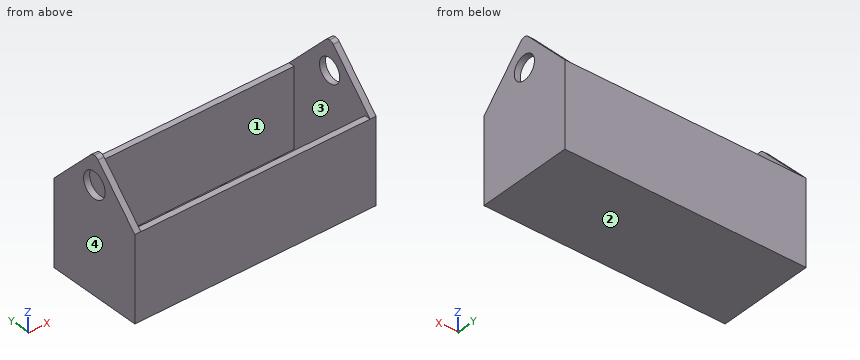
from build123d import *

# Parameters (mm, degrees)
F0_W      = 254
F0_H      = 101.6
F1_DEPTH  = 88.9
F4_DEPTH  = 6.35
F2_W      = 241.3
F2_H      = 88.9
F8_DEPTH  = 82.55
F9_R      = 12.7
F10_DEPTH = 25.4
F11_R     = 13.5154213428
F12_DEPTH = 25.4


with BuildPart() as f1:
    # F0 (on Top) → F1 (new body)
    with BuildSketch(Plane.XY):
        with Locations((77.3512227356, 27.0002914594)):
            Rectangle(F0_W, F0_H)
    extrude(amount=F1_DEPTH)

    # F3 (on face) → F4 (join)
    with BuildSketch(Plane.YZ.offset(204.3512227356)):
        with BuildLine():
            Line((22.3877730248, 137.7143067824), (-23.7997085406, 88.9))
            Line((-23.7997085406, 88.9), (27.0002914594, 88.9))
            Line((27.0002914594, 88.9), (27.0002914594, 139.7))
            ThreePointArc((27.0002914594, 139.7), (24.489399991, 139.1824886656), (22.3877730248, 137.7143067824))
        make_face()
        with BuildLine():
            Line((27.0002914594, 139.7), (27.0002914594, 88.9))
            Line((27.0002914594, 88.9), (77.8002914594, 88.9))
            Line((77.8002914594, 88.9), (31.6128098939, 137.7143067824))
            ThreePointArc((31.6128098939, 137.7143067824), (29.5111829277, 139.1824886656), (27.0002914594, 139.7))
        make_face()
    extrude(amount=-F4_DEPTH)

    # F7: F1 across plane


with BuildPart() as f1_1:
    add(f1.part)
    add(f1.part.mirror(Plane(origin=(77.3512227356, 27.0002914594, 88.9), x_dir=(0, 1, 0), z_dir=(1, 0, 0))))

    # F2 (on face) → F8 (cut)
    with BuildSketch(Plane.XY.offset(88.9)):
        with Locations((77.3512227356, 27.0002914594)):
            Rectangle(F2_W, F2_H)
    extrude(amount=-F8_DEPTH, mode=Mode.SUBTRACT)

    # F9 (on face) → F10 (cut)
    with BuildSketch(Plane.YZ.offset(204.3512227356)):
        with Locations((27.0002914594, 109.2127263546)):
            Circle(F9_R)
    extrude(amount=-F10_DEPTH, mode=Mode.SUBTRACT)

    # F11 (on face) → F12 (cut)
    with BuildSketch(Plane(origin=(-49.6487772644, 0, 0), x_dir=(0, -1, 0), z_dir=(-1, 0, 0))):
        with Locations((-27.0002914594, 110.0281476974)):
            Circle(F11_R)
    extrude(amount=-F12_DEPTH, mode=Mode.SUBTRACT)


solid = f1_1.part
Could you check a few things on this model? Use its own coordinates, in mm. Face numbers are marked on the shaded views. Give positions to 0.01 mm unless a question says otherwise; leave off trailing zeros. Order: outer loops, then holes, each group sorted by start corner. A loop starts at its lowest first (then second) coordinate and runs counter-clockwise, first axis right, second up. Notation, with made-up numbers: (69, 81) - (95, 81) arc R21 cw to (95, 120) - close; hole circle Ø5 at (-26, 60). An arc over 180 degrees is marked (long way). Return JSON: item names as keys, results as strings. Group by question number.
Q1. Suppose I cut it at B-B, the plane z = 99.5. Please give me the cut outline in (x, y), and give its area (3 significant figures).
Q2. Suppose I cut it at A-A, the plane z = 42.5. Please give me the cut outline in (x, y).
Q3. Suppose I cut it at D-D, the plane x = 182. Please give me the cut outline in (y, z), and give its area (3 significant figures).
Q4. Will these pins go through, and if not, where does the flat tip stop? pin 1 Ø1 at (x, y) = (53.5, -8) entering from +Z; pin 2 Ø1.9 at (x, y) = (121.5, 73) entering from +Z.
Q5. Suppose I cut it at C-C, the plane y = -8. Please give me the cut outline in (x, z), and give its area (3 significant figures).
Q6. Thinking about a two-plate mould opening in X: for the marked faces 1, 2, 3 and 4, which applies, pulls with the +X half, pulls with the -X half, needs draft (parallel to the pull), parting line crosses it, or undercut?
Q7. Please list where these lines run through material, in increasing order: line 1 along X through (y, z) = (32, 77.5); line 2 along Y through (x, z) = (164, 87); line 3 along Z through (x, y) = (94.5, 27.5). Write a range as [from, to].
Resolved:
{
 "1": {"outline": "(-49.65, -13.77) - (-43.3, -13.77) - (-43.3, 18.53) - (-49.65, 18.53) - close; (-49.65, 35.48) - (-43.3, 35.48) - (-43.3, 67.77) - (-49.65, 67.77) - close; (198, -13.77) - (204.35, -13.77) - (204.35, 18.82) - (198, 18.82) - close; (198, 35.18) - (204.35, 35.18) - (204.35, 67.77) - (198, 67.77) - close", "area": "824 mm2"},
 "2": {"outline": "(-49.65, -23.8) - (204.35, -23.8) - (204.35, 77.8) - (-49.65, 77.8) - close; hole (-43.3, -17.45) - (198, -17.45) - (198, 71.45) - (-43.3, 71.45) - close"},
 "3": {"outline": "(-23.8, 0) - (77.8, 0) - (77.8, 88.9) - (71.45, 88.9) - (71.45, 6.35) - (-17.45, 6.35) - (-17.45, 88.9) - (-23.8, 88.9) - close", "area": "1,690 mm2"},
 "4": {"pin 1": "stops at z = 6.35", "pin 2": "stops at z = 88.9"},
 "5": {"outline": "(-49.65, 0) - (204.35, 0) - (204.35, 105.6) - (198, 105.6) - (198, 6.35) - (-43.3, 6.35) - (-43.3, 105.6) - (-49.65, 105.6) - close", "area": "2,870 mm2"},
 "6": {"face 1": "undercut", "face 2": "needs draft", "face 3": "undercut", "face 4": "pulls with the -X half"},
 "7": {"line 1": "x = [-49.65, -43.3], [198, 204.35]", "line 2": "y = [-23.8, -17.45], [71.45, 77.8]", "line 3": "z = [0, 6.35]"}
}
